The listing builds one solid part. Answer for the finished solid, in the listing's coordinates (mm). A direction names the side the tool comes from. Round coordinates to 2 decimals unless told otherwise and drop trailing zeros. Loops run counter-clockwise (first coordinate to the right, second up) from the corner with the lowest first, then second, coordinate; pieces in that order, holes last. Notation, with made-up numbers: (35, 14) - (62, 14) arc R35 cw to (62, 48) - close; hole circle Ø7 at (74.25, 57.25). An arc over 180 degrees is marked (long way). One line per item, written item: value.
```python
from build123d import *

# Parameters (mm, degrees)
SALIENTE_EXTRUIR1_DEPTH = 3


with BuildPart() as part:
    # Croquis1 → Saliente-Extruir1 (new body)
    with BuildSketch(Plane(origin=(0, 0, 0), x_dir=(1, 0, 0), z_dir=(0, 1, 0))):
        with BuildLine():
            Line((-35.322649353, -4.523785763), (-29.713798408, 25.866039525))
            Line((-29.713798408, 25.866039525), (-35.221795469, 52.273603799))
            Line((-35.221795469, 52.273603799), (-36.45117663, 78.681168073))
            ThreePointArc((-36.45117663, 78.681168073), (-34.470773885, 85.134483293), (-28.840989272, 88.859103754))
            Line((-28.840989272, 88.859103754), (0, 95.923167849))
            Line((0, 95.923167849), (28.745582144, 88.873347738))
            ThreePointArc((28.745582144, 88.873347738), (34.369430491, 85.153487685), (36.353462125, 78.709215227))
            Line((36.353462125, 78.709215227), (35.159044734, 52.307970662))
            Line((35.159044734, 52.307970662), (29.69822954, 25.906726097))
            Line((29.69822954, 25.906726097), (35.352965357, -4.492390106))
            Line((35.352965357, -4.492390106), (36.368027066, -26.718230301))
            ThreePointArc((36.368027066, -26.718230301), (34.398862632, -33.147130574), (28.803795931, -36.875883169))
            Line((28.803795931, -36.875883169), (2.42535625, -43.470493089))
            ThreePointArc((2.42535625, -43.470493089), (0, -43.769068087), (-2.42535625, -43.470493089))
            Line((-2.42535625, -43.470493089), (-28.730703822, -36.894156196))
            ThreePointArc((-28.730703822, -36.894156196), (-34.320110297, -33.172996946), (-36.295781209, -26.755426116))
            Line((-36.295781209, -26.755426116), (-35.322649353, -4.523785763))
        make_face()
        Polygon((-3.75, 40.923167849), (-23.175796102, 36.165180269), (-32.691771262, 75.016772472), (-13.451535653, 79.72931046), align=None, mode=Mode.SUBTRACT)
        Polygon((13.453962591, 79.739018214), (3.75, 40.923167849), (23.155384938, 36.082606371), (32.856809939, 74.888306377), align=None, mode=Mode.SUBTRACT)
        Polygon((-3.75, 10.923167849), (-13.474641094, -27.975396528), (-32.877491097, -23.124684028), (-23.176066096, 15.681015978), align=None, mode=Mode.SUBTRACT)
        Polygon((3.75, 10.923167849), (23.449436749, 15.706069173), (32.88700521, -23.164643472), (13.451648888, -27.883427703), align=None, mode=Mode.SUBTRACT)
    extrude(amount=SALIENTE_EXTRUIR1_DEPTH)


solid = part.part
```
1) For faces 1 (the flat face through (13.46, 1.48, -13.28)), 2 (the flat face through (14.17, 1.48, -92.45)), 3 (the flat face through (35.853, 1.479, 15.45)), 4 (the flat face through (-35.828, 1.479, -65.293)), determine the directions among +Z, -Z, +X, -X, +Y, -Y from which every point of the face is accessible in a straight line to the end or side of a thin tool.
Final values:
face 1: +Y, -Y
face 2: -Z, +X, +Y, -Y
face 3: +X, +Y, -Y
face 4: -X, +Y, -Y
2) Consider L1, parallel to X at y = 0.1, z = 21; L2, parallel to Z at x = -22, y = 2.05; L3, parallel to Z at x = 21, y = 0.45. Determine where each line is inside the solid, lowest interval first.
Final values:
L1: -36.04 to -32.35, -11.73 to 11.73, 32.36 to 36.11
L2: -90.53 to -77.64, -36.45 to -15.39, 25.84 to 38.58
L3: -90.77 to -77.85, -36.62 to -15.11, 26.05 to 38.83
3) A cutting plane is placed at D-D on z = -83. Give the vertices of the cut face in (x, y).
Final values:
outline: (-35.69, 0) - (35.6, 0) - (35.6, 3) - (-35.69, 3) - close
4) A cutting plane is placed at B-B on z = -54.5. Give the vertices of the cut face in (x, y), and give its area (3 significant figures).
Final values:
outline: (-35.33, 0) - (-27.67, 0) - (-27.67, 3) - (-35.33, 3) - close; (-7.14, 0) - (7.14, 0) - (7.14, 3) - (-7.14, 3) - close; (27.76, 0) - (35.26, 0) - (35.26, 3) - (27.76, 3) - close
area: 88.3 mm2
5) A cutting plane is placed at C-C on x = 17. Give the vertices of the cut face in (y, z).
Final values:
outline: (0, -91.75) - (3, -91.75) - (3, -78.85) - (0, -78.85) - close; (0, -37.62) - (3, -37.62) - (3, -14.14) - (0, -14.14) - close; (0, 27.02) - (3, 27.02) - (3, 39.83) - (0, 39.83) - close
6) A cutting plane is placed at A-A on y = 1.45. Give the number of separate pieces and of enclosed holes in the cut face, and give its area (3 significant figures).
Final values:
separate pieces: 1
enclosed holes: 4
area: 5,780 mm2
7) For a pull along Z with two mould halves and no side action, classify faces 5 (the flat face through (-14.622, 1.479, -92.342)), 6 (the cylindrical face through (0.03, 1.48, 43.77)), 7 (the flat face through (-35.816, 1.479, 15.795)), 8 (the flat face through (32.467, 1.479, -39.292)) as released by +Z, released by -Z, zero draft, split by the parting line, or undercut.
Final values:
face 5: released by -Z
face 6: released by +Z
face 7: undercut
face 8: undercut
